Autodesk Fusion 360 part; units mm, degrees
sketch "Sketch1" plane through (0, 0, 0) normal (0, 0, 1) x (1, 0, 0)
  line L0 (0, 0) -> (-76.2, 0)
  line L1 (-76.2, 0) -> (-76.2, 76.2)
  line L2 (0, 76.2) -> (0, 0)
  line L3 (0, 76.2) -> (0, 88.9)
  line L4 (0, 88.9) -> (-76.2, 88.9)
  line L5 (-76.2, 88.9) -> (-76.2, 76.2)
  line L6 (-76.2, 0) -> (-63.5, 0)
  line L7 (-63.5, 0) -> (-63.5, -3.175)
  line L8 (-63.5, -3.175) -> (-50.8, -3.175)
  line L9 (-50.8, -3.175) -> (-50.8, 0)
  line L10 (-50.8, 0) -> (-38.1, 0)
  line L11 (0, 0) -> (-12.7, 0)
  line L12 (-12.7, 0) -> (-12.7, -3.175)
  line L13 (-12.7, -3.175) -> (-25.4, -3.175)
  line L14 (-25.4, -3.175) -> (-25.4, 0)
  line L15 (-76.2, 88.9) -> (-63.5, 88.9)
  line L16 (-63.5, 88.9) -> (-63.5, 92.075)
  line L17 (-63.5, 92.075) -> (-50.8, 92.075)
  line L18 (-50.8, 92.075) -> (-50.8, 88.9)
  line L19 (0, 88.9) -> (-12.7, 88.9)
  line L20 (-12.7, 88.9) -> (-12.7, 92.075)
  line L21 (-12.7, 92.075) -> (-25.4, 92.075)
  line L22 (-25.4, 92.075) -> (-25.4, 88.9)
  line L23 (-76.2, 0) -> (-76.2, 12.7)
  line L24 (-76.2, 12.7) -> (-79.375, 12.7)
  line L25 (-79.375, 12.7) -> (-79.375, 25.4)
  line L26 (-79.375, 25.4) -> (-76.2, 25.4)
  line L27 (-76.2, 88.9) -> (-76.2, 76.2)
  line L28 (-76.2, 76.2) -> (-79.375, 76.2)
  line L29 (-79.375, 76.2) -> (-79.375, 63.5)
  line L30 (-79.375, 63.5) -> (-76.2, 63.5)
  line L31 (3.175, 12.7) -> (3.175, 25.4)
  line L32 (3.175, 12.7) -> (0, 12.7)
  line L33 (3.175, 25.4) -> (0, 25.4)
  line L34 (0, 88.9) -> (0, 76.2)
  line L35 (0, 76.2) -> (3.175, 76.2)
  line L36 (3.175, 76.2) -> (3.175, 63.5)
  line L37 (3.175, 63.5) -> (0, 63.5)
  dimension "d1" = 76.2
  dimension "d2" = 76.2
  dimension "d3" = 12.7
  dimension "d4" = 3.175
  dimension "d5" = 12.7
  dimension "d6" = 12.7
  dimension "d7" = 12.7
  dimension "d8" = 3.175
  dimension "d9" = 12.7
  dimension "d10" = 12.7
  dimension "d11" = 3.175
  dimension "d12" = 12.7
  dimension "d13" = 12.7
  dimension "d14" = 3.175
  dimension "d15" = 12.7
  dimension "d16" = 12.7
  dimension "d17" = 3.175
  dimension "d18" = 12.7
  dimension "d19" = 12.7
  dimension "d20" = 3.175
  dimension "d21" = 12.7
  dimension "d24" = 12.7
  dimension "d25" = 12.7
  dimension "d26" = 3.175
  dimension "d27" = 12.7
extrude "Extrude1" add sketch "Sketch1" along normal blind 3.175
Can you work these out from the model? Positions are in its coordinate system, mm. A direction names the side the tool comes from. Coordinates: 2 decimals unless noted, no trailing zeros. Order: outer loops, then holes, each group sorted by start corner. A loop starts at its lowest first (then second) coordinate and runs counter-clockwise, first axis right, second up. Notation, with made-up numbers: (-16, -31) - (19, -31) arc R21 ccw to (19, -26) - close; hole circle Ø6 at (-40, 59.5). An arc over 180 degrees is marked (long way). Answer in a Markdown table with one row per item.
1. If we mould it in two halves opening along Y, with no side actions, what happens to faces 6 (the flat face through (-78, 25.4, 2)), 7 (the flat face through (-57, 92.075, 2)), 8 (the flat face through (-76.2, 83, 2)), 9 (the flat face through (-78, 63.5, 2))? For each: pulls with the +Y half, pulls with the -Y half, needs draft (parallel to the pull), parting line crosses it, or undercut.
Reply:
| item | result |
|---|---|
| face 6 | undercut |
| face 7 | pulls with the +Y half |
| face 8 | needs draft |
| face 9 | undercut |
2. Suppose I cut it at B-B (x = -70). Please give me the cut outline in (y, z) (3 decimals).
Reply:
| item | result |
|---|---|
| outline | (0, 0) - (88.9, 0) - (88.9, 3.175) - (0, 3.175) - close |
3. For faces 1 (the flat face through (-63.5, 90, 2)), 2 (the flat face through (-63.5, -2, 2)), 3 (the flat face through (-12.7, 90, 2)), 4 (the flat face through (-50.8, -2, 2)), 5 (the flat face through (-12.7, -2, 2)), which set-ups out of +Z, -Z, +X, -X, +Y, -Y let a thin tool reach every point of the face, with its end or its side?
Reply:
| item | result |
|---|---|
| face 1 | +Z, -Z, -X, +Y |
| face 2 | +Z, -Z, -X, -Y |
| face 3 | +Z, -Z, +X, +Y |
| face 4 | +Z, -Z, -Y |
| face 5 | +Z, -Z, +X, -Y |
4. If I drill on line 1 along Y through (x, z) = (-6, 1.65); line 2 along X through (y, z) = (87, 1), over which ranges is the centre line in solid material (lowest first)?
Reply:
| item | result |
|---|---|
| line 1 | y = 0 to 88.9 |
| line 2 | x = -76.2 to 0 |
5. For pin 1 (1 mm diameter, centred on y = 7, z = 1, fed in from -X); pin 2 (1.6 mm diameter, centred on y = -1.5, z = 1, fed in from -X); pin 3 (1.6 mm diameter, centred on x = -36.5, z = 1.5, fed in from +Y), each with a flat end and sliding along its axis, tell me the tip position at first contact or that it passes through.
Reply:
| item | result |
|---|---|
| pin 1 | stops at x = -76.2 |
| pin 2 | stops at x = -63.5 |
| pin 3 | stops at y = 88.9 |
6. Suppose I cut it at A-A (y = 9.5). Please give me the cut outline in (x, z) (3 decimals), and give its area (3 significant figures).
Reply:
| item | result |
|---|---|
| outline | (-76.2, 0) - (0, 0) - (0, 3.175) - (-76.2, 3.175) - close |
| area | 242 mm^2 |
